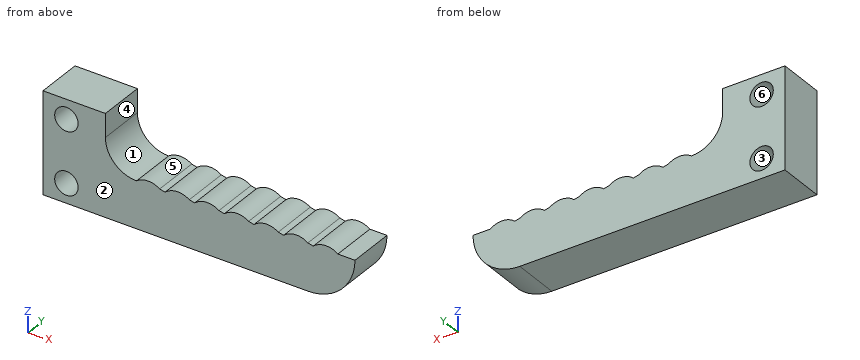
from build123d import *

# Parameters (mm, degrees)
BOSS_EXTRUDE1_DEPTH = 6
SKETCH2_R           = 1.5
CUT_EXTRUDE1_DEPTH  = 22.868927729


with BuildPart() as part:
    # Sketch1 → Boss-Extrude1 (new body)
    with BuildSketch(Plane.XZ):
        with BuildLine():
            Line((20, -0.5), (17.8, -0.5))
            ThreePointArc((17.8, -0.5), (16.025787821, -0.015083969), (14.4, -0.875192319))
            ThreePointArc((14.4, -0.875192319), (12.5, 0), (10.6, -0.875192319))
            ThreePointArc((10.6, -0.875192319), (8.7, 0), (6.8, -0.875192319))
            ThreePointArc((6.8, -0.875192319), (4.9, 0), (3, -0.875192319))
            ThreePointArc((3, -0.875192319), (1.1, 0), (-0.8, -0.875192319))
            ThreePointArc((-0.8, -0.875192319), (-2.7, 0), (-4.6, -0.875192319))
            ThreePointArc((-4.6, -0.875192319), (-6.225787821, -0.015083969), (-8, -0.5))
            ThreePointArc((-8, -0.5), (-10.828427125, 0.671572875), (-12, 3.5))
            Line((-12, 3.5), (-12, 6.5))
            Line((-12, 6.5), (-20, 6.5))
            Line((-20, 6.5), (-20, -6.5))
            Line((-20, -6.5), (14, -6.5))
            ThreePointArc((14, -6.5), (18.242640687, -4.742640687), (20, -0.5))
        make_face()
    extrude(amount=-BOSS_EXTRUDE1_DEPTH)

    # Chamfer1
    # the kernel refuses this chamfer: 0.5, 0.339586842 mm, written as the material it adds along each edge
    with BuildSketch(Plane(origin=(-4.6, 0, -0.875192319), x_dir=(0.7020641169662168, 0, 0.7121137378736954), z_dir=(0, 1, 0)), Plane(origin=(-0.8, 0, -0.875192319), x_dir=(0.7020641169662151, 0, 0.7121137378736971), z_dir=(0, 1, 0)), Plane(origin=(3, 0, -0.875192319), x_dir=(0.7020641169662145, 0, 0.7121137378736978), z_dir=(0, 1, 0)), Plane(origin=(6.8, 0, -0.875192319), x_dir=(0.7020641169662162, 0, 0.712113737873696), z_dir=(0, 1, 0)), Plane(origin=(10.6, 0, -0.875192319), x_dir=(0.7020641169662151, 0, 0.7121137378736971), z_dir=(0, 1, 0)), Plane(origin=(14.4, 0, -0.875192319), x_dir=(0.702064116966188, 0, 0.7121137378737239), z_dir=(0, 1, 0))) as chamfer1_piece_1:
        with BuildLine():
            Line((0.353747902, 0), (-0.021236492, -0.600134418))
            ThreePointArc((-0.021236492, -0.600134418), (0.007142061, -0.309444564), (0, 0))
            ThreePointArc((0, 0), (0.182204356, -0.006259046), (0.353747902, 0))
        make_face()
    extrude(amount=6)

    # Sketch2 → Cut-Extrude1 (cut, through all)
    with BuildSketch(Plane(origin=(0, 6, 0), x_dir=(1, 0, 0), z_dir=(0, 1, 0))):
        with Locations(Location((-17, 4, 0), (0, 0, 270))):
            Circle(SKETCH2_R)
        with Locations(Location((-17, -4, 0), (0, 0, 270))):
            Circle(SKETCH2_R)
    extrude(amount=-CUT_EXTRUDE1_DEPTH, mode=Mode.SUBTRACT)


solid = part.part
Can you work these out from the model? Positions are in its coordinate system, mm. Face numbers are marked on the shaded views. A direction names the side the tool comes from. Coordinates: 2 decimals unless noted, no trailing zeros. Loops run counter-clockwise (first coordinate to the right, second up) from the corner with the lowest first, then second, coordinate; pieces in that order, holes last. Notation, with made-up numbers: M 64.5,39.5 L 80.5,39.5 A10 ccw 80.5,55.5 Z; hole C 31.5,22 d3. An arc over 180 degrees is marked long. Return JSON: item names as keys, results as strings. Group by question number.
Item 1: Imagine slicing it at C-C (y = 4.6). Please give me the cut outline in (x, z), and give its area (3 significant figures).
Item 2: I'm going to push flat-ended pins straight in: pin 1 Ø1.8 at (x, z) = (-17, -4) entering from +Y; pin 2 Ø1.1 at (x, y) = (19.5, 3.5) entering from +Z; pin 3 Ø1.5 at (y, z) = (4, -4.5) entering from +X; pin 4 Ø0.9 at (y, z) = (2.5, 5) entering from +X. Where does each tip first touch, or does it pass through?
Item 3: If I drill on L1, parallel to X at y = 2.2, z = 4; L2, parallel to X at y = 4.3, z = 3.5; L3, parallel to Z at x = 14, y = 3.55, over which ranges is the centre line in solid material (lowest first)? Write a range as from..to.
Item 4: Imagine slicing it at B-B (z = 4). Please give me the cut outline in (x, y), and give its area (3 significant figures).
Item 5: Imagine slicing it at D-D (z = -3.75). Please give me the cut outline in (x, y), and give its area (3 significant figures).
Item 6: Thinking about a two-plate mould opening in Z: for the marked faces 3, 4, 5 and 6, which applies, released by +Z, released by -Z, zero draft, split by the parting line, or undercut?
Item 7: On a 3-axis mill with a long thin cutter (end or side, diameter ignored), from which of +Z, -Z, +X, -X, +Y, -Y can I reach the whole of each face in a straight line? I mean the marked faces 1 and 2. Say none if no direction works.
Item 8: Imagine slicing it at A-A (x = -17). Please give me the cut outline in (y, z), and give its area (3 significant figures).
Verdict:
{
 "1": {"outline": "M -20,-6.5 L 14,-6.5 A6 ccw 20,-0.5 L 17.8,-0.5 A2.5 ccw 14.65,-0.62 L 13.96,-0.47 A2.5 ccw 10.85,-0.62 L 10.16,-0.47 A2.5 ccw 7.05,-0.62 L 6.36,-0.47 A2.5 ccw 3.25,-0.62 L 2.56,-0.47 A2.5 ccw -0.55,-0.62 L -1.24,-0.47 A2.5 ccw -4.35,-0.62 L -5.04,-0.47 A2.5 ccw -8,-0.5 A4 cw -12,3.5 L -12,6.5 L -20,6.5 Z; hole C -17,-4 d3; hole C -17,4 d3", "area": "284 mm^2"},
 "2": {"pin 1": "passes through", "pin 2": "stops at z = -0.5", "pin 3": "stops at x = 19.04", "pin 4": "stops at x = -12"},
 "3": {"L1": "x = -20..-18.5, -15.5..-12", "L2": "x = -20..-18.41, -15.59..-12", "L3": "z = -6.5..-0.48"},
 "4": {"outline": "M -20,0 L -18.5,0 L -18.5,6 L -20,6 Z; M -15.5,0 L -12,0 L -12,6 L -15.5,6 Z", "area": "30.0 mm^2"},
 "5": {"outline": "M -20,0 L -18.48,0 L -18.48,6 L -20,6 Z; M -15.52,0 L 19.04,0 L 19.04,6 L -15.52,6 Z", "area": "217 mm^2"},
 "6": {"face 3": "undercut", "face 4": "zero draft", "face 5": "released by +Z", "face 6": "undercut"},
 "7": {"face 1": "+Z, +Y, -Y", "face 2": "+Z, -Z, +X, -X, -Y"},
 "8": {"outline": "M 0,-6.5 L 6,-6.5 L 6,-5.5 L 0,-5.5 Z; M 0,-2.5 L 6,-2.5 L 6,2.5 L 0,2.5 Z; M 0,5.5 L 6,5.5 L 6,6.5 L 0,6.5 Z", "area": "42.0 mm^2"}
}
